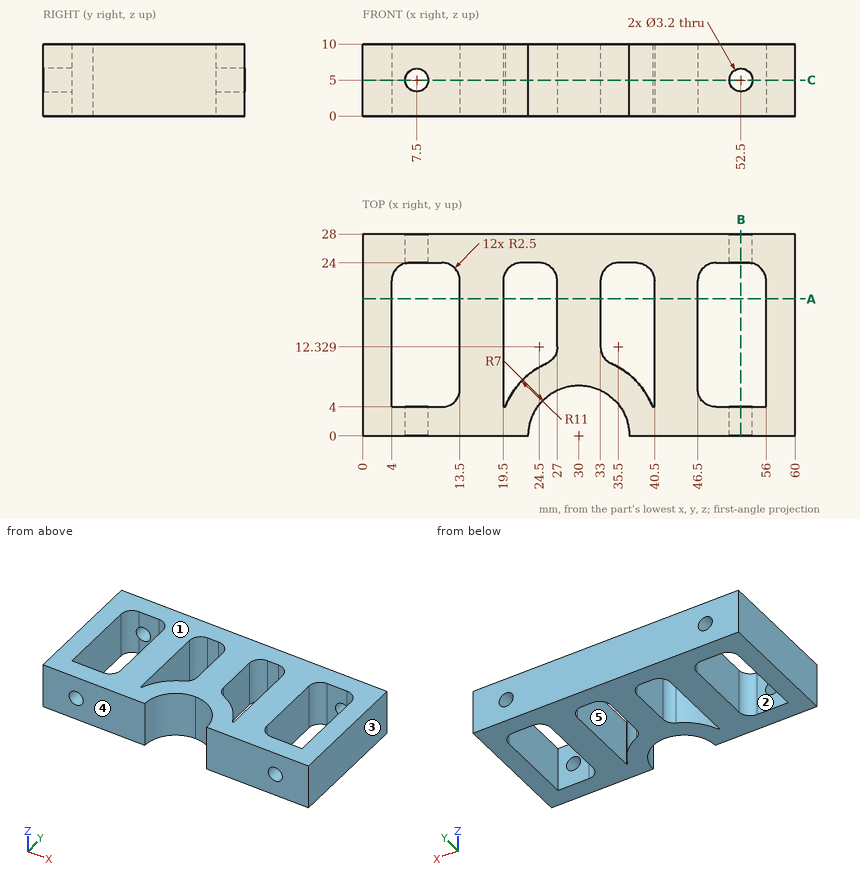
Design review of the part shown in the three views and the two pictorial views. Dimensions are in mm from the part's minimum x, y and z. A direction names the side the tool comes from. Give positions to 0.01 mm unless a question says otherwise; leave off trailing zeros. Write each loop counter-clockwise with the first axis right and the second up, starting at its lowest first coordinate (ties: lowest second). Pieces come first, ordered by that corner, then holes. Notation, with made-up numbers: (1.5, -32) - (35.5, -32) arc R17 cw to (35.5, -16) - close; hole circle Ø1 at (43.25, -38). An arc over 180 degrees is marked (long way). Return JSON: item names as keys, results as strings. Group by question number.
(1) Mouldability with a two-part tool opening along X and no side actions: class the marked faces 3, 4 and 5 as +X half, -X half, draft (parallel to the pull), parting line (faces both ways), or undercut.
(2) To check wall thickness, follow probe 1 along X at (y, z) = (26.25, 5); probe 2 along X at (y, z) = (12.5, 3.5); probe 3 along X at (y, z) = (8.5, 1.75). State the ranges of each line that lie inside material, in increasing order.
(3) We need section A-A, the plane y = 19. Give the boundary of the cut face in (x, z), then the cut area to 3 significant figures.
(4) We need section C-C, the plane z = 5. Give the number of separate pieces and of enclosed holes in the cut face, then the cut area to 3 significant figures.
(5) Machinability: for the marked faces 1 and 2, which of the approach directions +Z, -Z, +X, -X, +Y, -Y give a long, thin tool a straight path to every point of the face, cutting with its end or side? Answer none if there is none.
(6) Insertion check: pin 1 (2.5 mm diameter, centred on x = 7.5, z = 5, fed in from +Y). The pin has a flat end and moves straight along its axis. Give the tip position at first contact, or say it passes through.
(7) We need section B-B, the plane x = 52.5. Give the boundary of the cut face in (y, z).
Reported:
{
 "1": {"face 3": "+X half", "face 4": "draft", "face 5": "undercut"},
 "2": {"probe 1": "x = 0 to 5.9, 9.1 to 50.9, 54.1 to 60", "probe 2": "x = 0 to 4, 13.5 to 19.5, 27 to 33, 40.5 to 46.5, 56 to 60", "probe 3": "x = 0 to 4, 13.5 to 19.5, 23.02 to 36.98, 40.5 to 46.5, 56 to 60"},
 "3": {"outline": "(0, 0) - (4, 0) - (4, 10) - (0, 10) - close; (13.5, 0) - (19.5, 0) - (19.5, 10) - (13.5, 10) - close; (27, 0) - (33, 0) - (33, 10) - (27, 10) - close; (40.5, 0) - (46.5, 0) - (46.5, 10) - (40.5, 10) - close; (56, 0) - (60, 0) - (60, 10) - (56, 10) - close", "area": "260 mm2"},
 "4": {"separate pieces": "3", "enclosed holes": "2", "area": "949 mm2"},
 "5": {"face 1": "+Z, +X, -X, +Y, -Y", "face 2": "+Z, -Z"},
 "6": {"pin 1": "passes through"},
 "7": {"outline": "(0, 0) - (4, 0) - (4, 3.4) - (0, 3.4) - close; (0, 6.6) - (4, 6.6) - (4, 10) - (0, 10) - close; (24, 0) - (28, 0) - (28, 3.4) - (24, 3.4) - close; (24, 6.6) - (28, 6.6) - (28, 10) - (24, 10) - close"}
}
